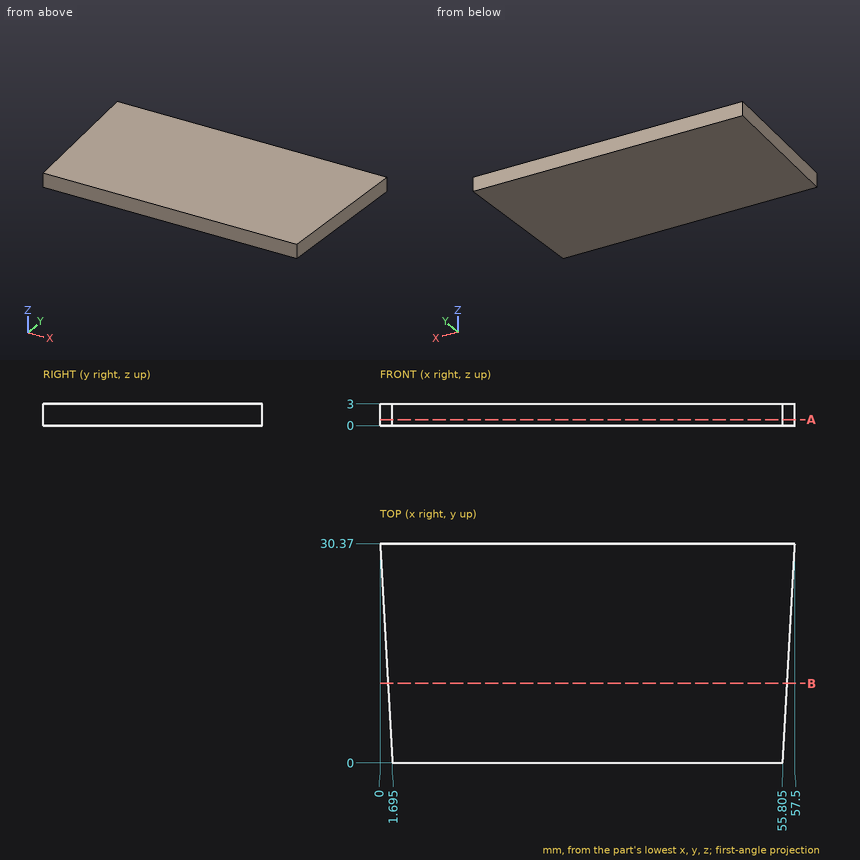
The drawing under review shows one solid part. Ordinate dimensions are in mm from its lowest x, y, z. Round coordinates to 2 decimals unless told otherwise and drop trailing zeros. Write each loop counter-clockwise with the first axis right and the second up, starting at its lowest first coordinate (ties: lowest second). Pieces come first, ordered by that corner, then holes. Notation, with made-up numbers: (83.25, 33) - (89.25, 33) arc R29 ccw to (89.25, 55) - close; hole circle Ø9 at (72, 82). An arc over 180 degrees is marked (long way). Put each result on its own line as item: value.
Q1. We need section A-A (z = 0.85). Give the boundary of the cut face in (x, y) (3 decimals), and give its area (3 significant figures).
Solved:
outline: (0, 30.37) - (1.695, 0) - (55.805, 0) - (57.5, 30.37) - close
area: 1,690 mm2
Q2. We need section B-B (y = 11). Give the boundary of the cut face in (x, z), and give its area (3 significant figures).
Solved:
outline: (1.08, 0) - (56.42, 0) - (56.42, 3) - (1.08, 3) - close
area: 166 mm2
Q3. Insertion check: pin 1 Ø1 at (x, z) = (8.5, 1) entering from -Y. The pin has a flat end and moves straight along its axis. Give the tip position at first contact, or say it passes through.
Solved:
pin 1: stops at y = 0
Q4. Wall thickness on probe 1 along X at (y, z) = (11, 0.35); probe 2 along X at (y, z) = (13.5, 2.9): over which ranges is each line inside the solid? List them lowest first.
Solved:
probe 1: x = 1.08 to 56.42
probe 2: x = 0.94 to 56.56
